Geometry: final body of the model. Coordinates: model frame, mm. Give positions to 0.01 mm unless a question says otherwise; leave off trailing zeros. Order: outer loops, then holes, each group sorted by start corner. A loop starts at its lowest first (then second) coordinate and runs counter-clockwise, first axis right, second up. Notation, with made-up numbers: M 44,14 L 58,14 A24 ccw 58,33 Z; hole C -17.5,-27.75 d4. An arc over 180 degrees is marked long. One line per item, written item: value. Start each with the question number.
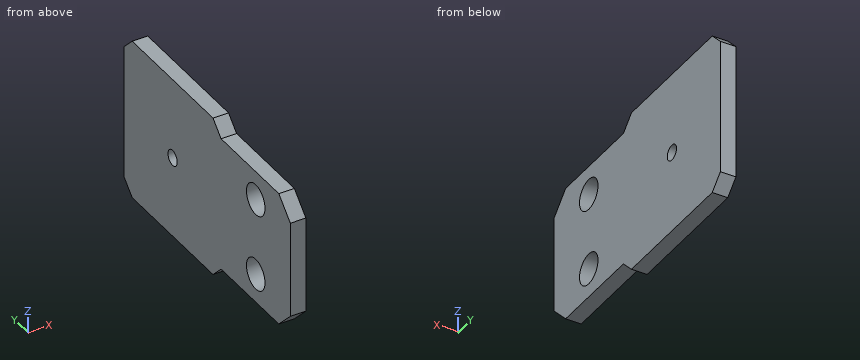
Autodesk Inventor part; units mm, degrees
ref_plane "YZ Plane" through (0, 0, 0) normal (1, 0, 0) x (0, 1, 0)
ref_plane "XZ Plane" through (0, 0, 0) normal (0, 1, 0) x (-1, 0, 0)
ref_plane "XY Plane" through (0, 0, 0) normal (0, 0, 1) x (1, 0, 0)
sketch "Эскиз1" plane through (0, 0, 0) normal (1, 0, 0) x (0, 1, 0)
  line L0 (-17.5, 21) -> (-21, 17.5)
  line L1 (-21, 17.5) -> (-21, -17.5)
  line L2 (-21, -17.5) -> (-17.5, -21)
  line L3 (-17.5, -21) -> (17.5, -21)
  line L4 (17.5, -21) -> (21, -17.5)
  line L5 (21, -17.5) -> (21, 17.5)
  line L6 (21, 17.5) -> (17.5, 21)
  line L7 (17.5, 21) -> (-17.5, 21)
  circle A0 centre (0, 0) radius 11.3
  line L8 (-21, 17.5) -> (-51, 17.5)
  line L9 (-51, 17.5) -> (-51, -17.5)
  line L10 (-51, -17.5) -> (-21, -17.5)
  line L11 (-21, -17.5) -> (-21, 17.5)
  line L12 (-51, 0) -> (-36, 0)
  line L13 (-36, 0) -> (-36, 10)
  line L14 (-36, 10) -> (-36, -10)
  circle A1 centre (-36, 10) radius 4
  circle A2 centre (-36, -10) radius 4
  circle A3 centre (0, 0) radius 2
  dimension "d0" = 30
  dimension "d1" = 15
  dimension "d2" = 10
  dimension "d3" = 20
  dimension "d4" = 8
  dimension "d5" = 8
  dimension "d6" = 4
extrude "Выдавливание1" add sketch "Эскиз1" along normal blind 4 contours L7 L6 L5 L4 L3 L2 L1 L0 | L1 L10 L9 L8 | A0
chamfer "Фаска1" distance 5 angle 45 2 edges at (2, -51, 17.5) (2, -51, -17.5)
properties part number "КВ33.044.002 - Держатель катка" material "Пластик АБС"
Q1. Section query D-D on z = -16. Return loops of the section in (x, y), and give its area (3 significant figures).
Q2. Section query B-B on y = -36. Return loops of the section in (x, z).
Q3. Contact query for flat-ended pins moving along their axis: pin 1 (6.5 mm diameter, centred on y = -36, z = 10, fed in from -X); pin 2 (2 mm diameter, centred on x = 1.5, y = -38, fed in from -Z); pin 3 (1.5 mm diameter, centred on x = 3, y = -33, fed in from +Z). Output: stop coordinate, or through.
Q4. Ray query, line 1 along Z through (x, y) = (1.7, -36); line 2 along Z through (x, y) = (0.65, -39); line 3 along Y through (x, z) = (0.9, 10). Return the intervals inside material, ascending. Write a range as [from, to].
Q5. Section query A-A on z = -10. Return loops of the section in (x, y).
Q6. Section query C-C on z = 0. Return loops of the section in (x, y).
Results below:
1. outline: M 0,-47.5 L 4,-47.5 L 4,21 L 0,21 Z
1. area: 274 mm2
2. outline: M 0,-17.5 L 4,-17.5 L 4,-14 L 0,-14 Z; M 0,-6 L 4,-6 L 4,6 L 0,6 Z; M 0,14 L 4,14 L 4,17.5 L 0,17.5 Z
3. pin 1: through
3. pin 2: z = -17.5
3. pin 3: z = 17.5
4. line 1: [-17.5, -14], [-6, 6], [14, 17.5]
4. line 2: [-17.5, -12.65], [-7.35, 7.35], [12.65, 17.5]
4. line 3: [-51, -40], [-32, 21]
5. outline: M 0,-51 L 4,-51 L 4,-40 L 0,-40 Z; M 0,-32 L 4,-32 L 4,21 L 0,21 Z
6. outline: M 0,-51 L 4,-51 L 4,-2 L 0,-2 Z; M 0,2 L 4,2 L 4,21 L 0,21 Z
